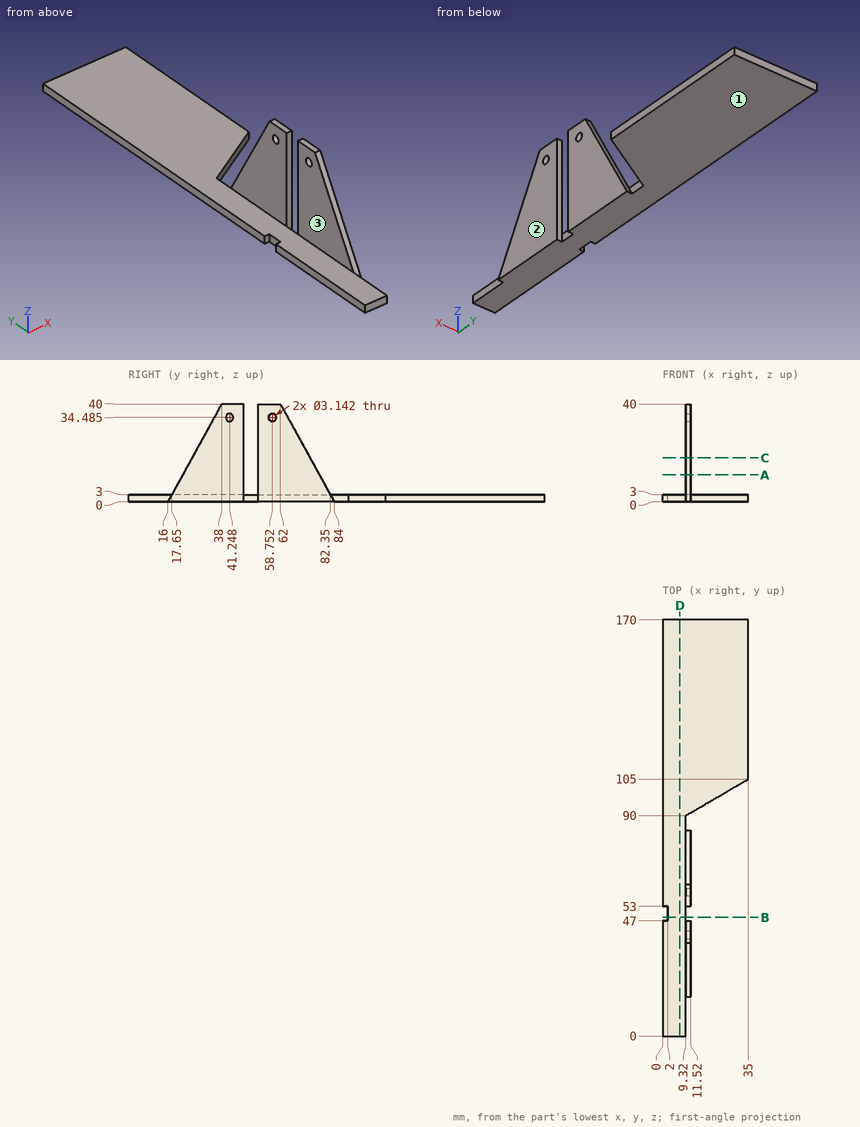
Could you check a few things on this drawing? It's one solid part, dimensions in mm from its lowest x, y, z. A direction names the side the tool comes from. Coordinates: 2 decimals unless noted, no trailing zeros. Loops run counter-clockwise (first coordinate to the right, second up) from the corner with the lowest first, then second, coordinate; pieces in that order, holes last. Notation, with made-up numbers: (-30.75, 47.5) - (19.25, 47.5) arc R12 cw to (19.25, 70.5) - close; hole circle Ø10 at (60, 18). An arc over 180 degrees is marked (long way). Return JSON: item names as keys, results as strings. Group by question number.
Item 1: If we section it at A-A on z = 11: Write out the boundary of the cut face in (x, y).
Item 2: Will these pins go through, and if not, where does the flat tip stop? P1, Ø14.5, axis at y = 71.5, z = 15.5, coming from the -X side; P2, Ø2.5, axis at y = 10, z = 2, coming from the +X side; P3, Ø9.5, axis at y = 64.5, z = 14, coming from the +X side.
Item 3: On a 3-axis mill with a long thin cutter (end or side, diameter ignored), from which of +Z, -Z, +X, -X, +Y, -Y can I reach the whole of each face in a straight line? I mean the marked faces 1, 2 and 3. Say none if no direction works.
Item 4: If we section it at D-D on x = 7: Write out the boundary of the cut face in (y, z).
Item 5: If we section it at B-B on y = 48.5: Write out the boundary of the cut face in (x, z).
Item 6: I need wall thicknesses on line 1 (X direction, y = 61.5, z = 2.5); line 2 (X direction, y = 58.5, z = 6.5); line 3 (Z direction, x = 9.5, y = 161). Which ranges of each line are inside material? Lowest first, please. Write a range as from..to.
Item 7: If we section it at C-C on z = 18: Write out the boundary of the cut face in (x, y).
Calculated:
{
 "1": {"outline": "(9.32, 22.05) - (11.52, 22.05) - (11.52, 47) - (9.32, 47) - close; (9.32, 53) - (11.52, 53) - (11.52, 77.95) - (9.32, 77.95) - close"},
 "2": {"P1": "stops at x = 9.32", "P2": "stops at x = 9.32", "P3": "stops at x = 11.52"},
 "3": {"face 1": "-Z, +X, -X, +Y, -Y", "face 2": "+Z, -Z, +X, -Y", "face 3": "+Z, -X, +Y, -Y"},
 "4": {"outline": "(0, 0) - (170, 0) - (170, 3) - (0, 3) - close"},
 "5": {"outline": "(2, 0) - (9.32, 0) - (9.32, 3) - (2, 3) - close"},
 "6": {"line 1": "x = 0..11.52", "line 2": "x = 9.32..11.52", "line 3": "z = 0..3"},
 "7": {"outline": "(9.32, 25.9) - (11.52, 25.9) - (11.52, 47) - (9.32, 47) - close; (9.32, 53) - (11.52, 53) - (11.52, 74.1) - (9.32, 74.1) - close"}
}
